from build123d import *

# Parameters (mm, degrees)
SKETCH_1_W      = 555
SKETCH_1_H      = 545
EXTRUDE_1_DEPTH = 580
SKETCH_2_W      = 595
SKETCH_2_H      = 595
EXTRUDE_2_DEPTH = 21
SKETCH_3_W      = 15
SKETCH_3_H      = 15
EXTRUDE_3_DEPTH = 30
SKETCH_4_W      = 465
SKETCH_4_H      = 15
EXTRUDE_4_DEPTH = 15


with BuildPart() as part:
    # Эскиз1 → Бобышка-Вытянуть1 (new body)
    with BuildSketch(Plane(origin=(0, 0, 0), x_dir=(1, 0, 0), z_dir=(0, 1, 0))):
        Rectangle(SKETCH_1_W, SKETCH_1_H)
    extrude(amount=EXTRUDE_1_DEPTH)

    # Эскиз2 → Бобышка-Вытянуть2 (add)
    with BuildSketch(Plane.XY.offset(272.5)):
        with Locations((0, 300.5)):
            Rectangle(SKETCH_2_W, SKETCH_2_H)
    extrude(amount=EXTRUDE_2_DEPTH)

    # Эскиз3 → Бобышка-Вытянуть3 (add)
    with BuildSketch(Plane.XY.offset(293.5)):
        with Locations((-225, 504.413440556)):
            Rectangle(SKETCH_3_W, SKETCH_3_H)
        with Locations((225, 504.413440556)):
            Rectangle(SKETCH_3_W, SKETCH_3_H)
    extrude(amount=EXTRUDE_3_DEPTH)

    # Эскиз4 → Бобышка-Вытянуть4 (add)
    with BuildSketch(Plane.XY.offset(323.5)):
        with Locations((0, 504.413440556)):
            Rectangle(SKETCH_4_W, SKETCH_4_H)
    extrude(amount=EXTRUDE_4_DEPTH)


solid = part.part
The model under review builds one solid part; all positions refer to its coordinate system, in mm. A direction names the side the tool comes from. Give positions to 0.01 mm unless a question says otherwise; leave off trailing zeros. Loops run counter-clockwise (first coordinate to the right, second up) from the corner with the lowest first, then second, coordinate; pieces in that order, holes last. Notation, with made-up numbers: (-37, 42.5) -> (8, 42.5) arc R26 cw to (8, 73.5) -> close; hole circle Ø10 at (89.25, 45.5). An arc over 180 degrees is marked (long way). Put each result on its own line as item: value. Start each with the question number.
1. Clearance check with flat-ended pins moving along their axes: P1, Ø3, axis at x = -51.5, z = 62.5, coming from the +Y side; P2, Ø12, axis at y = 502, z = 317.5, coming from the -X side; P3, Ø16.5, axis at y = 504, z = 308, coming from the +X side. State where each tip first meets the part, or that it passes through.
2. We need section A-A on x = -97. State the section outline as (y, z) points.
3. Wall thickness on probe 1 along X at (y, z) = (105.5, -101.5); probe 2 along Z at (x, y) = (126.5, 459); probe 3 along Y at (x, z) = (-79, 65): over which ranges is each line inside the solid? List them lowest first.
4. For faces 1 (the face through (-1, 496.913, 329)), 2 (the face through (277.5, 286, 4)), 3 (the face through (-277.5, 286, 4)), list the 3-axis set-ups (+Z, -Z, +X, -X, +Y, -Y) from which the entire face can be reached by the end or side of a thin tool; tool diameter is ignored.
5. We need section C-C on z = -207.5. State the section outline as (x, y) points.
6. We need section B-B on y = 136.5. State the section outline as (x, z) points, then the cut area to 3 significant figures.
Determined:
1. P1: y = 580
1. P2: x = -232.5
1. P3: x = 232.5
2. outline: (0, -272.5) -> (580, -272.5) -> (580, 272.5) -> (598, 272.5) -> (598, 293.5) -> (3, 293.5) -> (3, 272.5) -> (0, 272.5) -> close; (496.91, 323.5) -> (511.91, 323.5) -> (511.91, 338.5) -> (496.91, 338.5) -> close
3. probe 1: -277.5 to 277.5
3. probe 2: -272.5 to 293.5
3. probe 3: 0 to 580
4. face 1: +Z, +X, -X, -Y
4. face 2: -Z, +X, +Y, -Y
4. face 3: -Z, -X, +Y, -Y
5. outline: (-277.5, 0) -> (277.5, 0) -> (277.5, 580) -> (-277.5, 580) -> close
6. outline: (-297.5, 272.5) -> (-277.5, 272.5) -> (-277.5, -272.5) -> (277.5, -272.5) -> (277.5, 272.5) -> (297.5, 272.5) -> (297.5, 293.5) -> (-297.5, 293.5) -> close
6. area: 315,000 mm^2
